Geometry: final body of the model. Coordinates: model frame, mm. Face numbers are marked on the shaded views. Give positions to 0.01 mm unless a question says otherwise; leave off trailing zeros. Order: outer loops, then holes, each group sorted by start corner. A loop starts at its lowest first (then second) coordinate and runs counter-clockwise, first axis right, second up. Notation, with made-up numbers: M 57,-27 L 116,-27 A24 ccw 116,-9 Z; hole C 3,-26 d2. An arc over 180 degrees is marked long. Use CSV: the item, a comma, the result in double quotes.
Autodesk Fusion 360 part; units mm, degrees
sketch "Sketch1" plane through (0, 0, 0) normal (0, 1, 0) x (1, 0, 0)
  line L0 (0, 0) -> (125, 0)
  line L1 (125, 0) -> (125, -100)
  line L2 (125, -100) -> (0, -100)
  line L3 (0, -100) -> (0, 0)
  dimension "d1" = 125
  dimension "d2" = 100
extrude "Extrude1" add sketch "Sketch1" along normal blind 5
sketch "Sketch2" plane through (0, 5, 0) normal (0, 1, 0) x (-1, 0, 0)
  line L0 (0, 100) -> (-125, 100)
  line L1 (-125, 100) -> (-125, 0)
  line L2 (-125, 0) -> (0, 0)
  line L3 (0, 0) -> (0, 100)
  line L4 (-122, 3) -> (-3, 3)
  line L5 (-3, 3) -> (-3, 97)
  line L6 (-3, 97) -> (-122, 97)
  line L7 (-122, 97) -> (-122, 3)
  line L8 (-6, 6) -> (-59.3, 6)
  line L9 (-59.3, 6) -> (-59.3, 74.6)
  line L10 (-59.3, 74.6) -> (-6, 74.6)
  line L11 (-6, 74.6) -> (-6, 6)
  line L12 (-59.3, 6) -> (-52.3, 6)
  line L13 (-6, 6) -> (-37, 6)
  line L14 (-37, 3) -> (-52, 3)
  line L15 (-52, 3) -> (-52, 0)
  line L16 (-52, 0) -> (-37, 0)
  line L17 (-37, 0) -> (-37, 3)
  line L18 (-6, 6) -> (-6, 19.97)
  circle A0 centre (-8.54, 19.97) radius 1.5
  line L19 (-6, 6) -> (-6, 72.04)
  circle A1 centre (-13.62, 72.04) radius 1.65
  circle A2 centre (-41.56, 72.04) radius 1.65
  line L20 (-119, 6) -> (-64, 6)
  line L21 (-64, 6) -> (-64, 90)
  line L22 (-64, 90) -> (-119, 90)
  line L23 (-119, 90) -> (-119, 6)
  dimension "d9" = 53.3
  dimension "d10" = 68.6
  dimension "d11" = 7
  dimension "d12" = 31
  dimension "d13" = 13.97
  dimension "d14" = 2.54
  dimension "d15" = 3
  dimension "d16" = 66.04
  dimension "d17" = 7.62
  dimension "d18" = 35.56
  dimension "d19" = 3.3
  dimension "d20" = 3.3
  dimension "d21" = 55
  dimension "d22" = 84
extrude "Extrude2" cut sketch "Sketch2" against normal blind 5 contours A0 | A1 | A2
sketch "Sketch3" plane through (0, 5, 0) normal (0, 1, 0) x (-1, 0, 0)
  circle A0 centre (-8.54, 19.97) radius 1.5
  circle A1 centre (-13.62, 72.04) radius 1.65
  circle A2 centre (-41.56, 72.04) radius 1.65
  line L0 (0, 100) -> (-125, 100)
  line L1 (-125, 100) -> (-125, 0)
  line L2 (-125, 0) -> (0, 0)
  line L3 (0, 0) -> (0, 100)
  line L4 (-3, 3) -> (-123.5, 3)
  line L5 (-123.5, 3) -> (-123.5, 98.5)
  line L6 (-123.5, 98.5) -> (-3, 98.5)
  line L7 (-3, 98.5) -> (-3, 3)
  line L8 (-6, 6) -> (-59.3, 6)
  line L9 (-59.3, 6) -> (-59.3, 74.6)
  line L10 (-59.3, 74.6) -> (-6, 74.6)
  line L11 (-6, 74.6) -> (-6, 6)
  line L12 (-6, 6) -> (-37, 6)
  line L13 (-59.3, 6) -> (-51.3, 6)
  line L14 (-37, 3) -> (-51.3, 3)
  line L15 (-51.3, 3) -> (-51.3, 0)
  line L16 (-51.3, 0) -> (-37, 0)
  line L17 (-37, 0) -> (-37, 3)
  dimension "d25" = 53.3
  dimension "d26" = 68.6
  dimension "d27" = 31
  dimension "d28" = 8
extrude "Extrude3" add sketch "Sketch3" along normal blind 1 contours L0 L1 L2 L3 L4 L5 L6 L7 L15 L17
sketch "Sketch4" plane through (0, 0, 0) normal (0, -1, 0) x (1, 0, 0)
  circle A0 centre (8.54, 19.97) radius 1.5
  circle A1 centre (13.62, 72.04) radius 1.65
  circle A2 centre (41.56, 72.04) radius 1.65
  line L0 (125, 100) -> (0, 100)
  line L1 (0, 100) -> (0, 0)
  line L2 (0, 0) -> (125, 0)
  line L3 (125, 0) -> (125, 100)
  circle A3 centre (8.54, 19.97) radius 3.5
  circle A4 centre (13.62, 72.04) radius 3.5
  circle A5 centre (41.56, 72.04) radius 3.5
  dimension "d31" = 7
  dimension "d32" = 7
  dimension "d33" = 7
extrude "Extrude4" cut sketch "Sketch4" against normal blind 2.5 contours A3 | A4 | A5
extrude "Extrude5" add 1 faces at (1, 6, 34.3333) along direction (0, 1, 0) blind 17
sketch "Sketch5" plane through (0, 5, 0) normal (0, 1, 0) x (-1, 0, 0)
  line L0 (-51.3, 3) -> (-51.3, 0)
  line L1 (-51.3, 0) -> (-37, 0)
  line L2 (-37, 0) -> (-37, 3)
  line L3 (-37, 3) -> (-3, 3)
  line L4 (-3, 3) -> (-3, 98.5)
  line L5 (-3, 98.5) -> (-123.5, 98.5)
  line L6 (-123.5, 98.5) -> (-123.5, 3)
  line L7 (-123.5, 3) -> (-51.3, 3)
  circle A0 centre (-8.54, 19.97) radius 1.5
  circle A1 centre (-13.62, 72.04) radius 1.65
  circle A2 centre (-41.56, 72.04) radius 1.65
  line L8 (-51.3, 3) -> (-37, 3)
  line L9 (-37, 3) -> (-37, 0)
  line L10 (-37, 0) -> (-51.3, 0)
  line L11 (-51.3, 0) -> (-51.3, 3)
extrude "Extrude6" add sketch "Sketch5" along normal blind 0.4 contours L0 L1 L2 L8 L9 L10 L11
extrude "Extrude7" cut 1 faces at (1, 23, 34.3333) along direction (0, -1, 0) blind 2
sketch "Sketch6" plane through (0, 21, 0) normal (0, 1, 0) x (-1, 0, 0)
  line L0 (0, 0) -> (0, 100)
  line L1 (0, 100) -> (-125, 100)
  line L2 (-125, 100) -> (-125, 0)
  line L3 (-125, 0) -> (-51.3, 0)
  line L4 (-51.3, 0) -> (-51.3, 3)
  line L5 (-51.3, 3) -> (-123.5, 3)
  line L6 (-123.5, 3) -> (-123.5, 98.5)
  line L7 (-123.5, 98.5) -> (-3, 98.5)
  line L8 (-3, 98.5) -> (-3, 3)
  line L9 (-3, 3) -> (-37, 3)
  line L10 (-37, 3) -> (-37, 0)
  line L11 (-37, 0) -> (0, 0)
  line L12 (-37, 0) -> (-51.3, 0)
  line L13 (-51.3, 0) -> (-51.3, 3)
  line L14 (-51.3, 3) -> (-37, 3)
  line L15 (-37, 3) -> (-37, 0)
extrude "Extrude8" add sketch "Sketch6" along normal blind 44 contours L0 L1 L2 L3 L4 L5 L6 L7 L8 L9 L10 L11 L13 L15 | L4 L10 L12 L13 L14 L15
sketch "Sketch7" plane through (0, 0, 3) normal (0, 0, 1) x (1, 0, 0)
  line L0 (3, 65) -> (3, 5)
  line L1 (3, 5) -> (123.5, 5)
  line L2 (123.5, 5) -> (123.5, 65)
  line L3 (123.5, 65) -> (3, 65)
  line L4 (37, 21) -> (51.3, 21)
  line L5 (51.3, 21) -> (51.3, 5.4)
  line L6 (51.3, 5.4) -> (37, 5.4)
  line L7 (37, 5.4) -> (37, 21)
  circle A0 centre (60, 12) radius 5
  dimension "d44" = 10
extrude "Extrude9" cut sketch "Sketch7" against normal blind 3 contours A0
extrude "Extrude10" add 1 faces at (83.3333, 25, 98.5) along direction (0, 0, -1) blind 1.5
extrude "Extrude11" add 1 faces at (123.5, 25, 34.3333) along direction (-1, 0, 0) blind 1.5
sketch "Sketch8" plane through (0, 5, 0) normal (0, 1, 0) x (-1, 0, 0)
  line L0 (-122, 97) -> (-122, 3)
  line L1 (-122, 3) -> (-3, 3)
  line L2 (-3, 3) -> (-3, 97)
  line L3 (-3, 97) -> (-122, 97)
  circle A0 centre (-41.56, 72.04) radius 1.65
  circle A1 centre (-13.62, 72.04) radius 1.65
  circle A2 centre (-8.54, 19.97) radius 1.5
sketch "Sketch9" plane through (0, 65, 0) normal (0, 1, 0) x (-1, 0, 0)
  line L0 (-3, 3) -> (-122, 3)
  line L1 (-122, 3) -> (-122, 97)
  line L2 (-122, 97) -> (-3, 97)
  line L3 (-3, 97) -> (-3, 3)
  line L4 (0, 0) -> (0, 100)
  line L5 (0, 100) -> (-125, 100)
  line L6 (-125, 100) -> (-125, 0)
  line L7 (-125, 0) -> (0, 0)
  line L8 (-122, 97) -> (-112, 97)
  line L9 (-112, 97) -> (-112, 87)
  line L10 (-112, 87) -> (-122, 87)
  line L11 (-122, 87) -> (-122, 97)
  line L12 (-122, 3) -> (-112, 3)
  line L13 (-112, 3) -> (-112, 13)
  line L14 (-112, 13) -> (-122, 13)
  line L15 (-122, 13) -> (-122, 3)
  line L16 (-3, 97) -> (-13, 97)
  line L17 (-13, 97) -> (-13, 87)
  line L18 (-13, 87) -> (-3, 87)
  line L19 (-3, 87) -> (-3, 97)
  line L20 (-3, 3) -> (-13, 3)
  line L21 (-13, 3) -> (-13, 13)
  line L22 (-13, 13) -> (-3, 13)
  line L23 (-3, 13) -> (-3, 3)
  dimension "d51" = 10
  dimension "d52" = 10
  dimension "d53" = 10
  dimension "d54" = 10
  dimension "d55" = 10
  dimension "d56" = 10
extrude "Extrude12" add sketch "Sketch9" against normal blind 3 contours L0 L3 L20 L21 L22 L23 | L0 L1 L12 L13 L14 L15 | L2 L3 L16 L17 L18 L19 | L1 L2 L8 L9 L10 L11
sketch "Sketch10" plane through (0, 65, 0) normal (0, 1, 0) x (-1, 0, 0)
  line L0 (-13, 3) -> (-112, 3)
  line L1 (-112, 3) -> (-112, 13)
  line L2 (-112, 13) -> (-122, 13)
  line L3 (-122, 13) -> (-122, 87)
  line L4 (-122, 87) -> (-112, 87)
  line L5 (-112, 87) -> (-112, 97)
  line L6 (-112, 97) -> (-13, 97)
  line L7 (-13, 97) -> (-13, 87)
  line L8 (-13, 87) -> (-3, 87)
  line L9 (-3, 87) -> (-3, 13)
  line L10 (-3, 13) -> (-13, 13)
  line L11 (-13, 13) -> (-13, 3)
  line L12 (0, 0) -> (0, 100)
  line L13 (0, 100) -> (-125, 100)
  line L14 (-125, 100) -> (-125, 0)
  line L15 (-125, 0) -> (0, 0)
  circle A0 centre (-8, 8) radius 1.65
  circle A1 centre (-8, 92) radius 1.65
  circle A2 centre (-117, 92) radius 1.65
  circle A3 centre (-117, 8) radius 1.65
  dimension "d59" = 3.3
  dimension "d60" = 3.3
  dimension "d61" = 3.3
  dimension "d62" = 3.3
extrude "Extrude13" cut sketch "Sketch10" against normal blind 3 contours A0 | A1 | A2 | A3
delete_face "DeleteFace1" 1 faces at (115.3521, 63, 91.9178)
delete_face "DeleteFace2" 1 faces at (117.7527, 63, 6.5317)
delete_face "DeleteFace3" 2 faces at (6.3582, 64, 7.8357) (6.3521, 63, 91.9178)
sketch "Sketch11" plane through (0, 65, 0) normal (0, 1, 0) x (-1, 0, 0)
  line L0 (-13, 3) -> (-112, 3)
  line L1 (-112, 3) -> (-112, 13)
  line L2 (-112, 13) -> (-122, 13)
  line L3 (-122, 13) -> (-122, 87)
  line L4 (-122, 87) -> (-112, 87)
  line L5 (-112, 87) -> (-112, 97)
  line L6 (-112, 97) -> (-13, 97)
  line L7 (-13, 97) -> (-13, 87)
  line L8 (-13, 87) -> (-3, 87)
  line L9 (-3, 87) -> (-3, 13)
  line L10 (-3, 13) -> (-13, 13)
  line L11 (-13, 13) -> (-13, 3)
  line L12 (0, 0) -> (0, 100)
  line L13 (0, 100) -> (-125, 100)
  line L14 (-125, 100) -> (-125, 0)
  line L15 (-125, 0) -> (0, 0)
  line L16 (-13, 13) -> (-3, 13)
  line L17 (-3, 13) -> (-3, 3)
  line L18 (-3, 3) -> (-13, 3)
  line L19 (-13, 3) -> (-13, 13)
  line L20 (-13, 87) -> (-3, 87)
  line L21 (-3, 87) -> (-3, 97)
  line L22 (-3, 97) -> (-13, 97)
  line L23 (-13, 97) -> (-13, 87)
  line L24 (-112, 87) -> (-122, 87)
  line L25 (-122, 87) -> (-122, 97)
  line L26 (-122, 97) -> (-112, 97)
  line L27 (-112, 97) -> (-112, 87)
  line L28 (-112, 13) -> (-122, 13)
  line L29 (-122, 13) -> (-122, 3)
  line L30 (-122, 3) -> (-112, 3)
  line L31 (-112, 3) -> (-112, 13)
extrude "Extrude14" cut sketch "Sketch11" against normal blind 3 contours L10 L11 L16 L17 L18 L19 | L1 L2 L28 L29 L30 L31 | L7 L8 L20 L21 L22 L23 | L4 L5 L24 L25 L26 L27
sketch "Sketch12" plane through (0, 65, 0) normal (0, 1, 0) x (-1, 0, 0)
  line L0 (-3, 97) -> (-3, 3)
  line L1 (-3, 3) -> (-122, 3)
  line L2 (-122, 3) -> (-122, 97)
  line L3 (-122, 97) -> (-3, 97)
  line L4 (0, 0) -> (0, 100)
  line L5 (0, 100) -> (-125, 100)
  line L6 (-125, 100) -> (-125, 0)
  line L7 (-125, 0) -> (0, 0)
  line L8 (-3, 3) -> (-8, 3)
  line L9 (-8, 3) -> (-8, 8)
  line L10 (-8, 8) -> (-3, 8)
  line L11 (-3, 8) -> (-3, 3)
  line L12 (-3, 97) -> (-8, 97)
  line L13 (-8, 97) -> (-8, 92)
  line L14 (-8, 92) -> (-3, 92)
  line L15 (-3, 92) -> (-3, 97)
  line L16 (-122, 97) -> (-117, 97)
  line L17 (-117, 97) -> (-117, 92)
  line L18 (-117, 92) -> (-122, 92)
  line L19 (-122, 92) -> (-122, 97)
  line L20 (-122, 3) -> (-117, 3)
  line L21 (-117, 3) -> (-117, 8)
  line L22 (-117, 8) -> (-122, 8)
  line L23 (-122, 8) -> (-122, 3)
extrude "Extrude15" add sketch "Sketch12" against normal blind 5 contours L0 L3 L12 L13 L14 L15 | L0 L1 L8 L9 L10 L11 | L2 L3 L16 L17 L18 L19 | L1 L2 L20 L21 L22 L23
sketch "Sketch13" plane through (0, 65, 0) normal (0, 1, 0) x (-1, 0, 0)
  line L0 (-3, 92) -> (-3, 8)
  line L1 (-3, 8) -> (-8, 8)
  line L2 (-8, 8) -> (-8, 3)
  line L3 (-8, 3) -> (-117, 3)
  line L4 (-117, 3) -> (-117, 8)
  line L5 (-117, 8) -> (-122, 8)
  line L6 (-122, 8) -> (-122, 92)
  line L7 (-122, 92) -> (-117, 92)
  line L8 (-117, 92) -> (-117, 97)
  line L9 (-117, 97) -> (-8, 97)
  line L10 (-8, 97) -> (-8, 92)
  line L11 (-8, 92) -> (-3, 92)
  line L12 (0, 0) -> (0, 100)
  line L13 (0, 100) -> (-125, 100)
  line L14 (-125, 100) -> (-125, 0)
  line L15 (-125, 0) -> (0, 0)
  circle A0 centre (-5.5, 5.5) radius 1.65
  line L16 (-8, 92) -> (-5.5, 92)
  line L17 (-8, 94.5) -> (-8, 92)
  circle A1 centre (-5.5, 94.5) radius 1.65
  line L18 (-117, 92) -> (-119.5, 92)
  line L19 (-117, 94.5) -> (-117, 92)
  circle A2 centre (-119.5, 94.5) radius 1.65
  line L20 (-117, 8) -> (-119.5, 8)
  line L21 (-117, 5.5) -> (-117, 8)
  circle A3 centre (-119.5, 5.5) radius 1.65
  dimension "d69" = 3.3
  dimension "d70" = 3.3
  dimension "d71" = 3.3
  dimension "d72" = 3.3
extrude "Extrude16" cut sketch "Sketch13" against normal blind 5 contours A0 | A1 | A2 | A3
sketch "Sketch14" plane through (0, 65, 0) normal (0, 1, 0) x (-1, 0, 0)
  circle A0 centre (-119.5, 5.5) radius 1.65
  circle A1 centre (-5.5, 5.5) radius 1.65
  circle A2 centre (-119.5, 94.5) radius 1.65
  circle A3 centre (-5.5, 94.5) radius 1.65
  line L0 (-3, 92) -> (-3, 8)
  line L1 (-3, 8) -> (-8, 8)
  line L2 (-8, 8) -> (-8, 3)
  line L3 (-8, 3) -> (-117, 3)
  line L4 (-117, 3) -> (-117, 8)
  line L5 (-117, 8) -> (-122, 8)
  line L6 (-122, 8) -> (-122, 92)
  line L7 (-122, 92) -> (-117, 92)
  line L8 (-117, 92) -> (-117, 97)
  line L9 (-117, 97) -> (-8, 97)
  line L10 (-8, 97) -> (-8, 92)
  line L11 (-8, 92) -> (-3, 92)
  line L12 (0, 0) -> (0, 100)
  line L13 (0, 100) -> (-125, 100)
  line L14 (-125, 100) -> (-125, 0)
  line L15 (-125, 0) -> (0, 0)
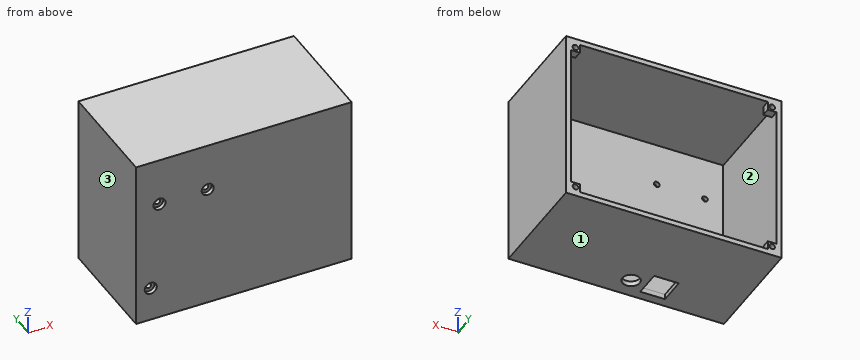
1. Section A-A, the plane z = 19.97. Return the cut outline in (x, y).
Answer:
outline,"M 0,0 L 5.04,0 L 5.04,2.5 L 7.04,2.5 L 7.04,5 L 3,5 L 3,65 L 0,65 Z; M 10.04,2.5 L 12.04,2.5 L 12.04,0 L 125,0 L 125,65 L 122,65 L 122,5 L 10.04,5 Z"
2. Section D-D, the plane y = 43. Return the cut outline in (x, z), plus the area to 3 significant figures.
Answer:
outline,"M 0,0 L 125,0 L 125,100 L 0,100 Z; hole M 3,3 L 122,3 L 122,97 L 3,97 Z"
area,"1,310 mm2"
3. Section C-C, the plane x = 41.56. Return the cut outline in (y, z), plus the area to 3 significant figures.
Answer:
outline,"M 0,0 L 5.4,0 L 5.4,3 L 5,3 L 5,70.39 L 2.5,70.39 L 2.5,68.54 L 0,68.54 Z; M 0,75.54 L 2.5,75.54 L 2.5,73.69 L 5,73.69 L 5,97 L 65,97 L 65,100 L 0,100 Z; M 21,0 L 65,0 L 65,3 L 21,3 Z"
area,"787 mm2"
4. Section B-B, the plane z = 94.5. Return the cut outline in (x, y), plus the area to 3 significant figures.
Answer:
outline,"M 0,0 L 125,0 L 125,65 L 121.15,65 L 121.15,60 L 122,60 L 122,5 L 3,5 L 3,60 L 3.85,60 L 3.85,65 L 0,65 Z; M 7.15,60 L 8,60 L 8,65 L 7.15,65 Z; M 117,60 L 117.85,60 L 117.85,65 L 117,65 Z"
area,"1,000 mm2"
5. Pull-direction query (X, two-part tool) for the marked faces 1, 2 and 3; classes: +X half, -X half, draft (parallel to the pull), parting line (faces both ways), or undercut.
Answer:
face 1,"draft"
face 2,"undercut"
face 3,"-X half"
6. Pin query (flat end, axial travel): pin 1 Ø1 at (x, z) = (104, 62.5) entering from +Y. Return the tip coordinate at first contact, or that it passes through.
Answer:
pin 1,"y = 5"
7. Line query: line 1 (X direction, y = 3.3, z = 72.04); line 2 (X direction, y = 62.6, z = 94.5); line 3 (Z direction, x = 5.5, y = 18). Output: solid intervals per line, ascending.
Answer:
line 1,"0 to 11.97, 15.27 to 39.91, 43.21 to 125"
line 2,"0 to 3.85, 7.15 to 8, 117 to 117.85, 121.15 to 125"
line 3,"0 to 3, 97 to 100"
